Input: part model. Units: mm. Frame: model coordinates. A direction names the side the tool comes from. Round coordinates to 2 decimals unless told otherwise and drop trailing zeros. Write each loop counter-clockwise with the first axis right and the second up, starting at its lowest first coordinate (ties: lowest second). Pieces come first, ordered by that corner, then holes. Notation, with made-up numbers: M -34,-17.5 L 22,-17.5 A30 ccw 22,6.5 Z; hole C 7.25,-21.5 d9. An arc over 180 degrees is marked long. Write each question's results on one line, items separated by ' | '. Start each with the question number.
```python
from build123d import *

# Parameters (mm, degrees)
CROQUIS1_R              = 5.5
SALIENTE_EXTRUIR1_DEPTH = 12


with BuildPart() as part:
    # Croquis1 → Saliente-Extruir1 (new body)
    with BuildSketch(Plane.XY):
        with BuildLine():
            Line((-181.041600866, 72.635135135), (-134.541600866, 72.635135135))
            ThreePointArc((-134.541600866, 72.635135135), (-131.041600866, 72.635135135), (-131.041600866, 76.135135135))
            Line((-131.041600866, 76.135135135), (-131.041600866, 90.635135135))
            Line((-131.041600866, 90.635135135), (-81.041600866, 90.635135135))
            Line((-81.041600866, 90.635135135), (-81.041600866, 76.135135135))
            ThreePointArc((-81.041600866, 76.135135135), (-81.041600866, 72.635135135), (-77.541600866, 72.635135135))
            Line((-77.541600866, 72.635135135), (-34.541600866, 72.635135135))
            ThreePointArc((-34.541600866, 72.635135135), (-31.041600866, 72.635135135), (-31.041600866, 76.135135135))
            Line((-31.041600866, 76.135135135), (-31.041600866, 90.635135135))
            Line((-31.041600866, 90.635135135), (18.958399134, 90.635135135))
            Line((18.958399134, 90.635135135), (18.958399134, 76.135135135))
            ThreePointArc((18.958399134, 76.135135135), (18.958399134, 72.635135135), (22.458399134, 72.635135135))
            Line((22.458399134, 72.635135135), (46.849903851, 72.635135135))
            ThreePointArc((46.849903851, 72.635135135), (50.494893062, 71.270913441), (50.958399134, 75.135135135))
            Line((50.958399134, 75.135135135), (50.958399134, 89.635135135))
            Line((50.958399134, 89.635135135), (100.958399134, 89.635135135))
            Line((100.958399134, 89.635135135), (100.958399134, 75.135135135))
            ThreePointArc((100.958399134, 75.135135135), (101.421905205, 71.270913441), (105.066894417, 72.635135135))
            Line((105.066894417, 72.635135135), (146.746184683, 72.635135135))
            ThreePointArc((146.746184683, 72.635135135), (150.038647504, 70.053679014), (150.958399134, 74.135135135))
            Line((150.958399134, 74.135135135), (150.958399134, 88.635135135))
            Line((150.958399134, 88.635135135), (200.958399134, 88.635135135))
            Line((200.958399134, 88.635135135), (200.958399134, 74.135135135))
            ThreePointArc((200.958399134, 74.135135135), (201.878150764, 70.053679014), (205.170613584, 72.635135135))
            Line((205.170613584, 72.635135135), (250.958399134, 72.635135135))
            Line((250.958399134, 72.635135135), (250.958399134, 8.635135135))
            Line((250.958399134, 8.635135135), (43.458399134, 8.635135135))
            Line((43.458399134, 8.635135135), (43.458399134, 20.635135135))
            ThreePointArc((43.458399134, 20.635135135), (41.115253383, 26.291989385), (35.458399134, 28.635135135))
            Line((35.458399134, 28.635135135), (-12.541600866, 28.635135135))
            ThreePointArc((-12.541600866, 28.635135135), (-18.198455116, 26.291989385), (-20.541600866, 20.635135135))
            Line((-20.541600866, 20.635135135), (-20.541600866, 8.635135135))
            Line((-20.541600866, 8.635135135), (-181.041600866, 8.635135135))
            Line((-181.041600866, 8.635135135), (-181.041600866, 72.635135135))
        make_face()
        with Locations((-156.041600866, 22.135135135)):
            Circle(CROQUIS1_R, mode=Mode.SUBTRACT)
        with Locations((225.958399134, 22.135135135)):
            Circle(CROQUIS1_R, mode=Mode.SUBTRACT)
    extrude(amount=SALIENTE_EXTRUIR1_DEPTH)


solid = part.part
```
1. Line query: L1, parallel to X at y = 78, z = 11.75; L2, parallel to X at y = 70.5, z = 7.5; L3, parallel to X at y = 20, z = 9.5. Output: solid intervals per line, ascending. Write a range as from..to.
2. Access query for faces 1 (the face through (-131.042, 83, 6)), 2 (the face through (228, 72.635, 6)), 3 (the face through (149, 8.635, 6)), 4 (the face through (100.958, 82, 6)), 5 (the face through (43.458, 15, 6)). Directions: +Z, -Z, +X, -X, +Y, -Y. A direction counts if a zero-diameter tool reaches every point of the face in a straight line with its end or side. Return the directions, or none.
3. Cut plane C-C on z = 7.5. Give the number of separate pieces and of enclosed holes in the cut face, and give its area (3 significant figures).
4. Draft query along X for faces 6 (the face through (250.958, 41, 6)), 7 (the face through (-106, 90.635, 6)), 8 (the face through (41.177, 26.229, 5.916)). Return one class per face: +X half, -X half, draft (parallel to the pull), parting line (faces both ways), or undercut.
5. Cut plane D-D on x = 124. Output: boundary loops of the cut face in (y, z), and give its area (3 significant figures).
6. Cut plane B-B on x = 182. Output: boundary loops of the cut face in (y, z).
7. Cut plane A-A on y = 83. Output: boundary loops of the cut face in (x, z), and give its area (3 significant figures).
8. Contact query for flat-ended pins moving along their axis: P1, Ø6, axis at x = 179.5, z = 5, coming from the +Y side; P2, Ø6, axis at y = 84.5, z = 4, coming from the +X side; P3, Ø2, axis at x = 201, y = 58, coming from the -Z side; P4, Ø6, axis at y = 84, z = 6.5, coming from the -X side. Output: stop coordinate, or through.
Answers follow:
1) L1: x = -131.04..-81.04, -31.04..18.96, 50.96..100.96, 150.96..200.96 | L2: x = -181.04..147.6, 150.81..201.1, 204.31..250.96 | L3: x = -181.04..-161.11, -150.97..-20.54, 43.46..220.89, 231.03..250.96
2) face 1: +Z, -Z, -X, +Y | face 2: +Z, -Z, +X, +Y | face 3: +Z, -Z, +X, -X, -Y | face 4: +Z, -Z, +Y | face 5: +Z, -Z, -Y
3) separate pieces: 1 | enclosed holes: 2 | area: 29,600 mm2
4) face 6: +X half | face 7: draft | face 8: undercut
5) outline: M 8.64,0 L 72.64,0 L 72.64,12 L 8.64,12 Z | area: 768 mm2
6) outline: M 8.64,0 L 88.64,0 L 88.64,12 L 8.64,12 Z
7) outline: M -131.04,0 L -81.04,0 L -81.04,12 L -131.04,12 Z; M -31.04,0 L 18.96,0 L 18.96,12 L -31.04,12 Z; M 50.96,0 L 100.96,0 L 100.96,12 L 50.96,12 Z; M 150.96,0 L 200.96,0 L 200.96,12 L 150.96,12 Z | area: 2,400 mm2
8) P1: stops at y = 88.64 | P2: stops at x = 200.96 | P3: stops at z = 0 | P4: stops at x = -131.04
